Can you work these out from the model? Positions are in its coordinate system, mm. Face numbers are marked on the shaded views. Give positions to 0.01 mm unless a question says otherwise; leave off trailing zeros. Order: outer loops, then holes, each group sorted by start corner. A loop starts at its lowest first (then second) coordinate and runs counter-clockwise, first axis right, second up. Notation, with made-up numbers: M 77,80 L 135,80 A25 ccw 135,116 Z; hole C 44.5,48 d5. An arc over 180 degrees is marked long. Use one line per item in the form item = value. Start each with the question number.
1. Will this pin go through, and if not, where does the flat tip stop? P1, Ø2, axis at x = -469.5, z = 73, coming from the -Y side.
2. I want a section at A-A, the plane y = -312. List the corners of the cut face in (x, z) for me, and give its area (3 significant figures).
3. I want a section at C-C, the plane x = 496.5. List the corners of the cut face in (y, z) for me (3 decimals), and give its area (3 significant figures).
4. I need wall thicknesses on L1, parallel to Y at x = 101.5, z = 117.5 (3 decimals); L2, parallel to Y at x = -208.5, z = -28 (3 decimals); L3, parallel to Y at x = 301, z = -468.5 (3 decimals). Which ranges of each line are inside material? Lowest first, please.
5. I want a section at B-B, the plane z = -393.5. List the corners of the cut face in (x, y) for me (3 decimals), and give its area (3 significant figures).
6. We'd pull the mould along Y, two halves only. Please class the marked faces 1 and 2: +Y half, -Y half, draft (parallel to the pull), parting line (faces both ways), or undercut.
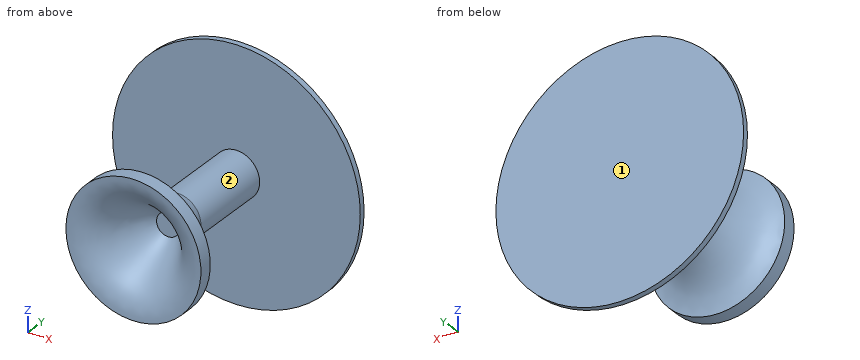
```python
from build123d import *

# Parameters (mm, degrees)
SKETCH2_W = 609.6
SKETCH2_H = 28.575


with BuildPart() as part:
    # Sketch2 → Revolve1 (revolve)
    with BuildSketch(Plane.XY, mode=Mode.PRIVATE) as revolve1_sk:
        Polygon((114.390414377, 0), (0, 0), (0, -508), (57.195207189, -508), (114.390414377, -508), (114.390414377, -436.856929751), align=None)
        with Locations((304.8, 14.2875)):
            Rectangle(SKETCH2_W, SKETCH2_H)
        with BuildLine():
            add(Edge.make_bspline(
                [(114.390414377, -436.856929751), (144.884830942, -546.818476347), (207.101707678, -672.816275805), (332.316500716, -696.853289197)],
                knots=[0, 0, 0, 0, 1, 1, 1, 1], degree=3))
            Line((114.390414377, -436.856929751), (114.390414377, -508))
            Line((114.390414377, -508), (57.195207189, -508))
            add(Edge.make_bspline(
                [(332.316500716, -766.703289197), (180.787832632, -766.227742439), (148.104498186, -589.357090779), (57.195207189, -508)],
                knots=[0, 0, 0, 0, 1, 1, 1, 1], degree=3))
            Line((332.316500716, -766.703289197), (332.316500716, -696.853289197))
        make_face()
    revolve(revolve1_sk.sketch.rotate(Axis((0, 0, 0), (0, -1, 0)), 180), axis=Axis((0, 0, 0), (0, -1, 0)))


solid = part.part
```
Check result:
q1.P1 = 0
q2.outline = C 0,0 d228.78
q2.area = 41,100 mm2
q3.outline = M 0,-353.695 L 28.575,-353.695 L 28.575,353.695 L 0,353.695 Z
q3.area = 20,200 mm2
q4.L1 = -642.803 to -545.142, 0 to 28.575
q4.L2 = -714.114 to -626.702, 0 to 28.575
q4.L3 = 0 to 28.575
q5.outline = M -465.586,0 L 465.586,0 L 465.586,28.575 L -465.586,28.575 Z
q5.area = 26,600 mm2
q6.face_1 = +Y half
q6.face_2 = undercut
